Geometry: see drawing. Coordinates: mm, zero at the bounding-box minimum. Round coordinates to 2 decimals unless told otherwise and drop trailing zeros. Write each loop counter-clockwise with the first axis right and the second up, starting at its lowest first coordinate (ties: lowest second). Pieces come first, ordered by that corner, then holes. Notation, with made-up numbers: M 14.25,60.25 L 33.25,60.25 A12 cw 33.25,82.25 Z; hole C 54,-8 d2. An arc over 180 degrees is marked long. Use one line per item in the form item = value. Start each with the question number.
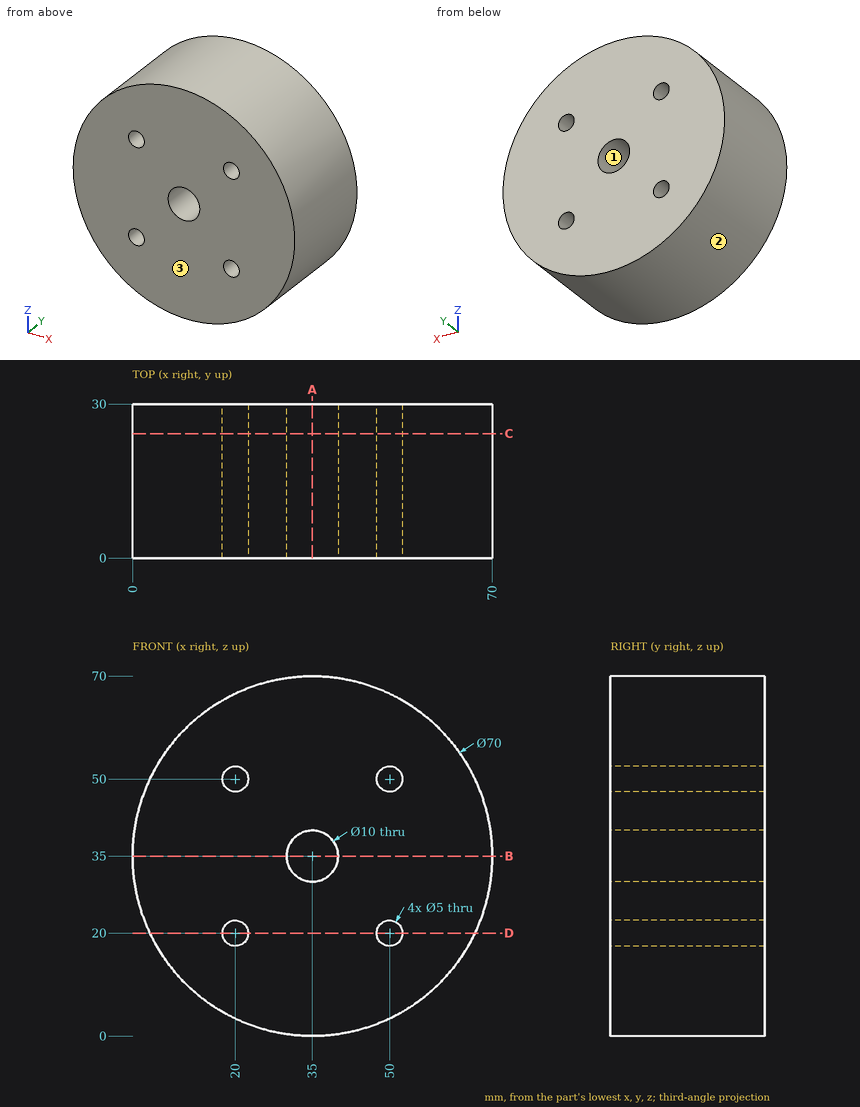
Item 1: Ray query, line 1 (Z direction, x = 50, y = 13.5); line 2 (Z direction, x = 35, y = 21); line 3 (Z direction, x = 21, y = 27.5). Return the intervals inside material, ascending. Write a range as from..to.
Item 2: Cut plane C-C (y = 24.25). Output: boundary loops of the cut face in (x, z).
Item 3: Cut plane A-A (x = 35). Output: boundary loops of the cut face in (y, z).
Item 4: Cut plane D-D (z = 20). Output: boundary loops of the cut face in (x, y), plus the area to 3 significant figures.
Item 5: Draft query along Z for the marked faces 1, 2 and 3. Return one class per face: +Z half, -Z half, draft (parallel to the pull), parting line (faces both ways), or undercut.
Item 6: Cut plane B-B (z = 35). Output: boundary loops of the cut face in (x, y).
Item 7: First-contact query: pin 1 (4.5 mm diameter, centred on x = 20, z = 20, fed in from +Y); pin 2 (3 mm diameter, centred on y = 6, z = 39.5, fed in from -X); pin 3 (5 mm diameter, centred on y = 6, z = 63, fed in from -X); pin 4 (6 mm diameter, centred on y = 11.5, z = 8, fed in from -X). Flat tips, straight axial feed; report the tip coordinate or a pass-through.
Final values:
q1.line_1 = 3.38..17.5, 22.5..47.5, 52.5..66.62
q1.line_2 = 0..30, 40..70
q1.line_3 = 2.92..17.71, 22.29..47.71, 52.29..67.08
q2.outline = C 35,35 d70; hole C 20,20 d5; hole C 20,50 d5; hole C 35,35 d10; hole C 50,20 d5; hole C 50,50 d5
q3.outline = M 0,0 L 30,0 L 30,30 L 0,30 Z; M 0,40 L 30,40 L 30,70 L 0,70 Z
q4.outline = M 3.38,0 L 17.5,0 L 17.5,30 L 3.38,30 Z; M 22.5,0 L 47.5,0 L 47.5,30 L 22.5,30 Z; M 52.5,0 L 66.62,0 L 66.62,30 L 52.5,30 Z
q4.area = 1,600 mm^2
q5.face_1 = undercut
q5.face_2 = parting line
q5.face_3 = draft
q6.outline = M 0,0 L 30,0 L 30,30 L 0,30 Z; M 40,0 L 70,0 L 70,30 L 40,30 Z
q7.pin_1 = through
q7.pin_2 = 0.13
q7.pin_3 = 11.03
q7.pin_4 = 9.52
